```python
from build123d import *

# Parameters (mm, degrees)
F0_W     = 180
F0_H     = 20
F1_DEPTH = 20
F3_DEPTH = 25
F4_R     = 2


with BuildPart() as f1:
    # F0 (on Front) → F1 (new body)
    with BuildSketch(Plane.XZ):
        with Locations((90, 10)):
            Rectangle(F0_W, F0_H)
    extrude(amount=-F1_DEPTH)

    # F2 (on face) → F3 (cut)
    with BuildSketch(Plane.XZ):
        with BuildLine():
            Line((75.7071421427, 20), (4.2928578573, 20))
            ThreePointArc((4.2928578573, 20), (40, 5), (75.7071421427, 20))
        make_face()
        with BuildLine():
            Line((175.7071421427, 20), (104.2928578573, 20))
            ThreePointArc((104.2928578573, 20), (140, 5), (175.7071421427, 20))
        make_face()
    extrude(amount=-F3_DEPTH, mode=Mode.SUBTRACT)

    # F4
    f4_edges = [f1.edges().sort_by_distance(p)[0] for p in [
        (0, 10, 20),
        (4.292858, 10, 20),
        (75.707142, 10, 20),
        (104.292858, 10, 20),
        (175.707142, 10, 20),
        (180, 10, 20),
    ]]
    fillet(f4_edges, radius=F4_R)


solid = f1.part
```
Here's how the part is built. I have some questions about the finished solid (model axes, mm). Round coordinates to 2 decimals unless told otherwise and drop trailing zeros. Order: outer loops, then holes, each group sorted by start corner. A loop starts at its lowest first (then second) coordinate and runs counter-clockwise, first axis right, second up. Notation, with made-up numbers: M 68.25,32 L 99.25,32 A18 ccw 99.25,49 Z; hole C -37.75,23.5 d4. An arc over 180 degrees is marked long. One line per question, with ' | ' between items.
1) For pin 1 Ø12 at (x, y) = (28.5, 3) entering from +Z; pin 2 Ø4 at (x, z) = (22, 12) entering from +Y; pin 3 Ø12 at (x, y) = (153.5, 2.5) entering from +Z, each with a flat end and sliding along its axis, tell me the tip position at first contact or that it passes through.
Working result:
pin 1: z = 8.16 | pin 2: through | pin 3: z = 8.96
2) I want a section at A-A, the plane y = 12.25. Write out the boundary of the cut face in (x, z).
Working result:
outline: M 0,0 L 180,0 L 180,18 A2 ccw 178,20 L 176.54,20 A2 ccw 175.13,19.42 A50 cw 104.87,19.42 A2 ccw 103.46,20 L 76.54,20 A2 ccw 75.13,19.42 A50 cw 4.87,19.42 A2 ccw 3.46,20 L 2,20 A2 ccw 0,18 Z
3) If we mould it in two halves opening along X, with no side actions, what happens to faces 1 (the face through (39.455, 9.86, 5.003)), 2 (the face through (180, 10, 9)), 3 (the face through (89, 10, 0))? For each: +X half, -X half, draft (parallel to the pull), parting line (faces both ways), or undercut.
Working result:
face 1: undercut | face 2: +X half | face 3: draft
4) I want a section at D-D, the plane z = 9.5. Write out the boundary of the cut face in (x, y), then the cut area to 3 significant figures.
Working result:
outline: M 0,0 L 19.27,0 L 19.27,20 L 0,20 Z; M 60.73,0 L 119.27,0 L 119.27,20 L 60.73,20 Z; M 160.73,0 L 180,0 L 180,20 L 160.73,20 Z | area: 1,940 mm²
5) I want a section at B-B, the plane z = 16.25. Write out the boundary of the cut face in (x, y), then the cut area to 3 significant figures.
Working result:
outline: M 0,0 L 8.4,0 L 8.4,20 L 0,20 Z; M 71.6,0 L 108.4,0 L 108.4,20 L 71.6,20 Z; M 171.6,0 L 180,0 L 180,20 L 171.6,20 Z | area: 1,070 mm²
6) I want a section at C-C, the plane x = 110. Write out the boundary of the cut face in (y, z), then the cut area to 3 significant figures.
Working result:
outline: M 0,0 L 20,0 L 20,15 L 0,15 Z | area: 300 mm²
7) I need wall thicknesses on line 1 along X through (y, z) = (3, 10.5); line 2 along X through (y, z) = (6.75, 11.25); line 3 along Z through (x, y) = (139, 1.5). Which ranges of each line are inside material? Lowest first, please.
Working result:
line 1: 0 to 17.2, 62.8 to 117.2, 162.8 to 180 | line 2: 0 to 15.79, 64.21 to 115.79, 164.21 to 180 | line 3: 0 to 5.01
